from build123d import *

# Parameters (mm, degrees)
SKETCH1_R           = 50
SKETCH1_R_2         = 35
BOSS_EXTRUDE1_DEPTH = 40
SKETCH2_W           = 120
SKETCH2_H           = 120
BOSS_EXTRUDE2_DEPTH = 5
SKETCH3_R           = 3
CUT_EXTRUDE1_DEPTH  = 5


with BuildPart() as part:
    # Sketch1 → Boss-Extrude1 (new body)
    with BuildSketch(Plane(origin=(0, 0, 0), x_dir=(1, 0, 0), z_dir=(0, 1, 0))):
        with Locations(Location((0, 0, 0), (0, 0, 270))):
            Circle(SKETCH1_R)
        with Locations(Location((0, 0, 0), (0, 0, 270))):
            Circle(SKETCH1_R_2, mode=Mode.SUBTRACT)
    extrude(amount=BOSS_EXTRUDE1_DEPTH)

    # Sketch2 → Boss-Extrude2 (add)
    with BuildSketch(Plane(origin=(0, 0, 0), x_dir=(1, 0, 0), z_dir=(0, 1, 0))):
        Rectangle(SKETCH2_W, SKETCH2_H)
    extrude(amount=BOSS_EXTRUDE2_DEPTH)

    # Sketch3 → Cut-Extrude1 (cut)
    with BuildSketch(Plane(origin=(0, 5, 0), x_dir=(1, 0, 0), z_dir=(0, 1, 0))):
        with Locations(Location((-50, 50, 0), (0, 0, 270))):
            Circle(SKETCH3_R)
        with Locations(Location((50, -50, 0), (0, 0, 270))):
            Circle(SKETCH3_R)
    extrude(amount=-CUT_EXTRUDE1_DEPTH, mode=Mode.SUBTRACT)


solid = part.part
CAD build for the part. Positions are in the model's coordinates, mm. A direction names the side the tool comes from. Coordinates: 2 decimals unless noted, no trailing zeros. Write each loop counter-clockwise with the first axis right and the second up, starting at its lowest first coordinate (ties: lowest second). Pieces come first, ordered by that corner, then holes. Notation, with made-up numbers: (-1.75, -1.5) - (39.25, -1.5) arc R28 cw to (39.25, 24.5) - close; hole circle Ø5 at (12.25, 22.5). An arc over 180 degrees is marked (long way). Use a Markdown table: item, result. Add a question column.
Item 1: Band-saw the part on A-A, the plane z = 0. Give the cut face in (x, y).
Item 2: Drill centre lines: L1, parallel to X at y = 31, z = 0; L2, parallel to X at y = 1, z = 50. Where is each one in solid material? Low to high. Write a range as from..to.
Item 3: Band-saw the part on B-B, the plane x = 0. Give the cut face in (y, z).
Item 4: Flat gauge pins, fed straight in: pin 1 (4 mm diameter, centred on x = -32, z = 31.5, fed in from -Y); pin 2 (1 mm diameter, centred on y = 21.5, z = -29.5, fed in from -X); pin 3 (4 mm diameter, centred on y = 11, z = 11, fed in from +X); pin 4 (12 mm diameter, centred on y = 20, z = 18.5, fed in from -X). Where does each tip first touch, or does it go through?
Item 5: 3-axis set-ups, long thin cutter, end or side, ignore diameter. For faces 1 (the face through (52.03, 2.54, 47.79)), 2 (the face through (15.02, 22.26, 47.69)): which of +Z, -Z, +X, -X, +Y, -Y reach the whole face in a straight line?
Item 6: Band-saw the part on C-C, the plane x = -51.5. Give the cut face in (y, z).
Item 7: Band-saw the part on D-D, the plane y = 30. Give the cut face in (x, z).
Item 8: Mould opens along X. For faces 3 (the face through (60, 2, 1)), 4 (the face through (-1, 2, 60)), 5 (the face through (-21, 22, -28)) say: pulls with the +X half, pulls with the -X half, needs draft (parallel to the pull), parting line crosses it, or undercut.
Numbers:
| question | item | result |
|---|---|---|
| 1 | outline | (-60, 0) - (60, 0) - (60, 5) - (50, 5) - (50, 40) - (35, 40) - (35, 5) - (-35, 5) - (-35, 40) - (-50, 40) - (-50, 5) - (-60, 5) - close |
| 2 | L1 | -50..-35, 35..50 |
| 2 | L2 | -60..47, 53..60 |
| 3 | outline | (0, -60) - (5, -60) - (5, -50) - (40, -50) - (40, -35) - (5, -35) - (5, 35) - (40, 35) - (40, 50) - (5, 50) - (5, 60) - (0, 60) - close |
| 4 | pin 1 | y = 0 |
| 4 | pin 2 | x = -40.73 |
| 4 | pin 3 | x = 49.18 |
| 4 | pin 4 | x = -48.41 |
| 5 | face 1 | +Y, -Y |
| 5 | face 2 | +Y |
| 6 | outline | (0, -60) - (5, -60) - (5, -52.6) - (0, -52.6) - close; (0, -47.4) - (5, -47.4) - (5, 60) - (0, 60) - close |
| 7 | outline | circle Ø100 at (0, 0); hole circle Ø70 at (0, 0) |
| 8 | face 3 | pulls with the +X half |
| 8 | face 4 | needs draft |
| 8 | face 5 | undercut |
